from build123d import *

# Parameters (mm, degrees)
SKETCH_W        = 27
SKETCH_H        = 27
PAD_DEPTH       = 3
SKETCH001_W     = 16.4
SKETCH001_H     = 3
POCKET_DEPTH    = 5
SKETCH002_W     = 16.4
SKETCH002_H     = 11
POCKET001_DEPTH = 1.8
CHAMFER_SIZE    = 0.6
SKETCH003_R     = 2
POCKET002_DEPTH = 3.001


with BuildPart() as part:
    # Sketch → Pad (new body)
    with BuildSketch(Plane.XY):
        Rectangle(SKETCH_W, SKETCH_H)
    extrude(amount=PAD_DEPTH)

    # Sketch001 (on Face5 of Pad) → Pocket (cut)
    with BuildSketch(Plane(origin=(0, 0, 0), x_dir=(1, 0, 0), z_dir=(0, 0, -1))):
        with Locations((0, -6.7)):
            Rectangle(SKETCH001_W, SKETCH001_H)
    extrude(amount=-POCKET_DEPTH, mode=Mode.SUBTRACT)

    # Sketch002 (on Face4 of Pocket) → Pocket001 (cut)
    with BuildSketch(Plane(origin=(0, 0, 0), x_dir=(1, 0, 0), z_dir=(0, 0, -1))):
        with Locations((0, 2.3)):
            Rectangle(SKETCH002_W, SKETCH002_H)
    extrude(amount=-POCKET001_DEPTH, mode=Mode.SUBTRACT)

    # Chamfer
    chamfer_edges = [part.edges().sort_by_distance(p)[0] for p in [
        (8.2, -2.3, 0),
        (0, -7.8, 0),
        (-8.2, -2.3, 0),
        (0, 3.2, 0),
        (0, 5.2, 0),
        (8.2, 6.7, 0),
        (0, 8.2, 0),
        (-8.2, 6.7, 0),
    ]]
    chamfer(chamfer_edges, length=CHAMFER_SIZE)

    # Sketch003 (on Face18 of Chamfer) → Pocket002 (cut, through all)
    with BuildSketch(Plane.XY.offset(3)):
        with Locations((-10.1, 0.5)):
            Circle(SKETCH003_R)
        with Locations((10.1, 0.5)):
            Circle(SKETCH003_R)
    extrude(amount=-POCKET002_DEPTH, mode=Mode.SUBTRACT)


solid = part.part
Source: CAD feature listing. Evaluate the final solid. Frame: model axes, mm. A direction names the side the tool comes from. Coordinates: 2 decimals unless noted, no trailing zeros. Write each loop counter-clockwise with the first axis right and the second up, starting at its lowest first coordinate (ties: lowest second). Pieces come first, ordered by that corner, then holes. Notation, with made-up numbers: M 30.25,21.5 L 71.25,21.5 A7 ccw 71.25,26.5 Z; hole C 32,23.25 d8. An arc over 180 degrees is marked long. Use a Markdown table: item, result.
1) Section A-A, the plane x = -10.1. Output: boundary loops of the cut face in (y, z).
Conclusion:
| item | result |
|---|---|
| outline | M -13.5,0 L -1.5,0 L -1.5,3 L -13.5,3 Z; M 2.5,0 L 13.5,0 L 13.5,3 L 2.5,3 Z |
2) Mould query, pull axis Y, two halves, no side actions, for faces 1 (the flat face through (0, 13.5, 1)), 2 (the flat face through (8.2, 2, 1)), 3 (the flat face through (0, -13.5, 1)), 4 (the flat face through (0, 0, 3)). Classes: pulls with the +Y half, pulls with the -Y half, needs draft (parallel to the pull), parting line crosses it, or undercut.
Conclusion:
| item | result |
|---|---|
| face 1 | pulls with the +Y half |
| face 2 | undercut |
| face 3 | pulls with the -Y half |
| face 4 | needs draft |
3) Reachability of faces 5 (the flat face through (-8.2, 7, 2)), 6 (the flat face through (0, -7.8, 1)), 7 (the flat face through (0, 9, 0)) from +Z, -Z, +X, -X, +Y, -Y: full face, straight path, thin tool, end or side. Return the list, or none.
Conclusion:
| item | result |
|---|---|
| face 5 | +Z, -Z |
| face 6 | -Z |
| face 7 | -Z, +X, -X, +Y, -Y |
4) Ray query, L1, parallel to X at y = 0.5, z = 1.85; L2, parallel to Y at x = -2.25, z = 2.75; L3, parallel to Y at x = 10.1, z = 1.8. Return the intervals inside material, ascending.
Conclusion:
| item | result |
|---|---|
| L1 | x = -13.5 to -12.1, -8.1 to 8.1, 12.1 to 13.5 |
| L2 | y = -13.5 to 5.2, 8.2 to 13.5 |
| L3 | y = -13.5 to -1.5, 2.5 to 13.5 |
5) First-contact query: pin 1 Ø12 at (x, y) = (-0.5, -4) entering from -Z. Flat tip, straight axial feed; report the tip coordinate or a pass-through.
Conclusion:
| item | result |
|---|---|
| pin 1 | stops at z = 0 |
6) Section B-B, the plane y = 0.5. Output: boundary loops of the cut face in (x, z), then the cut area to 3 significant figures.
Conclusion:
| item | result |
|---|---|
| outline | M -13.5,0 L -12.1,0 L -12.1,3 L -13.5,3 Z; M -8.1,1.8 L 8.1,1.8 L 8.1,3 L -8.1,3 Z; M 12.1,0 L 13.5,0 L 13.5,3 L 12.1,3 Z |
| area | 27.8 mm^2 |
7) Section C-C, the plane x = -1. Output: boundary loops of the cut face in (y, z).
Conclusion:
| item | result |
|---|---|
| outline | M -13.5,0 L -8.4,0 L -7.8,0.6 L -7.8,1.8 L 3.2,1.8 L 3.2,0.6 L 3.8,0 L 4.6,0 L 5.2,0.6 L 5.2,3 L -13.5,3 Z; M 8.2,0.6 L 8.8,0 L 13.5,0 L 13.5,3 L 8.2,3 Z |
